Work out the finished part from the listing and answer in its coordinate system (mm). Face numbers are marked on the shaded views. Coordinates: 2 decimals unless noted, no trailing zeros. Order: outer loops, then holes, each group sorted by start corner. A loop starts at its lowest first (then second) coordinate and runs counter-clockwise, first axis right, second up. Notation, with made-up numbers: (69, 41) -> (99, 41) arc R22 ccw to (99, 58) -> close; hole circle Ø5 at (11, -20). An arc over 180 degrees is marked (long way). Write item = value, one per line. Start each with the question number.
Q1. The part is cut by section C-C, the plane y = 3.5. Determine the outline of the cut face in (x, z), plus the area to 3 significant figures.
Q2. Straight lines are drawn through the part: L1, parallel to Z at x = 0, y = -1; L2, parallel to X at y = -2.3, z = 0; L3, parallel to Y at x = 41, z = -18. For each, find the intervals that lie inside material, in ascending order. Write a range as from..to.
Q3. For a pull along X with two mould halves and no side action, classify the marked faces 1, 2 and 3 as +X half, -X half, draft (parallel to the pull), parting line (faces both ways), or undercut.
Q4. The part is cut by section B-B, the plane y = 93. Determine the outline of the cut face in (x, z), plus the area to 3 significant figures.
Q5. Flat-ended cylindrical pins translate along their axes: pin 1 (4 mm diameter, centred on y = 9.5, z = 1, fed in from +X); pin 2 (6 mm diameter, centred on x = -67.5, z = 82, fed in from +Y); pin 3 (1 mm diameter, centred on x = -48, z = -69.5, fed in from +Y); pin 4 (8 mm diameter, centred on x = -71.5, z = 87.5, fed in from +Y). Find the tip coordinate at first contact, or state that the pin passes through.
Q6. The part is cut by section A-A, the plane z = 0. Determine the outline of the cut face in (x, y).
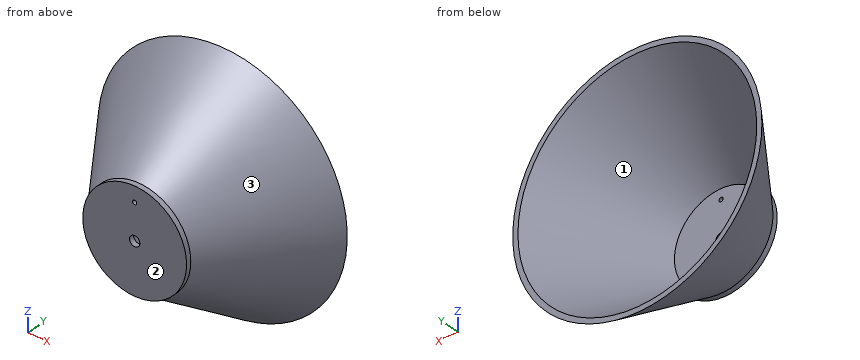
Autodesk Inventor part; units mm, degrees
ref_plane "YZ Plane" through (0, 0, 0) normal (1, 0, 0) x (0, 1, 0)
ref_plane "XZ Plane" through (0, 0, 0) normal (0, 1, 0) x (-1, 0, 0)
ref_plane "XY Plane" through (0, 0, 0) normal (0, 0, 1) x (1, 0, 0)
sketch "Szkic6" plane through (0, 0, 0) normal (0, 1, 0) x (-1, 0, 0)
  circle A0 centre (0, 0) radius 50
  dimension "d28" = 100
extrude "Wyciągnięcie proste5" add sketch "Szkic6" along normal blind 100 draft 35
sketch "Szkic7" plane through (0, 0, 0) normal (0, -1, 0) x (1, 0, 0)
  circle A0 centre (0, 0) radius 45
  dimension "d31" = 90
extrude "Wyciągnięcie proste6" cut sketch "Szkic7" against normal blind 100 draft 35
sketch "Szkic8" plane through (0, 0, 0) normal (0, -1, 0) x (1, 0, 0)
  circle A0 centre (0, 0) radius 50
extrude "Wyciągnięcie proste7" add sketch "Szkic8" along normal blind 5
sketch "Szkic9" plane through (0, -5, 0) normal (0, -1, 0) x (1, 0, 0)
  circle A0 centre (0, 35) radius 2
  point P0 (0, 0)
  dimension "d36" = 4
extrude "Wyciągnięcie proste8" cut sketch "Szkic9" against normal blind 5
sketch "Szkic10" plane through (0, 0, 0) normal (0, 1, 0) x (1, 0, 0)
  circle A0 centre (0, 0) radius 5
  dimension "d39" = 10
extrude "Wyciągnięcie proste9" cut sketch "Szkic10" against normal blind 5
properties part number "Lejek"
Model answer:
q1.outline = circle Ø104.9 at (0, 0); hole circle Ø94.9 at (0, 0)
q1.area = 1,570 mm2
q2.L1 = -50..-5, 5..33, 37..50
q2.L2 = -50..-5, 5..50
q2.L3 = -5..0
q3.face_1 = undercut
q3.face_2 = draft
q3.face_3 = parting line
q4.outline = circle Ø230.24 at (0, 0); hole circle Ø220.24 at (0, 0)
q4.area = 3,540 mm2
q5.pin_1 = 58.04
q5.pin_2 = 91.7
q5.pin_3 = 57.08
q5.pin_4 = 100
q6.outline = (-120.02, 100) -> (-50, 0) -> (-50, -5) -> (-5, -5) -> (-5, 0) -> (-45, 0) -> (-115.02, 100) -> close; (5, -5) -> (50, -5) -> (50, 0) -> (120.02, 100) -> (115.02, 100) -> (45, 0) -> (5, 0) -> close
